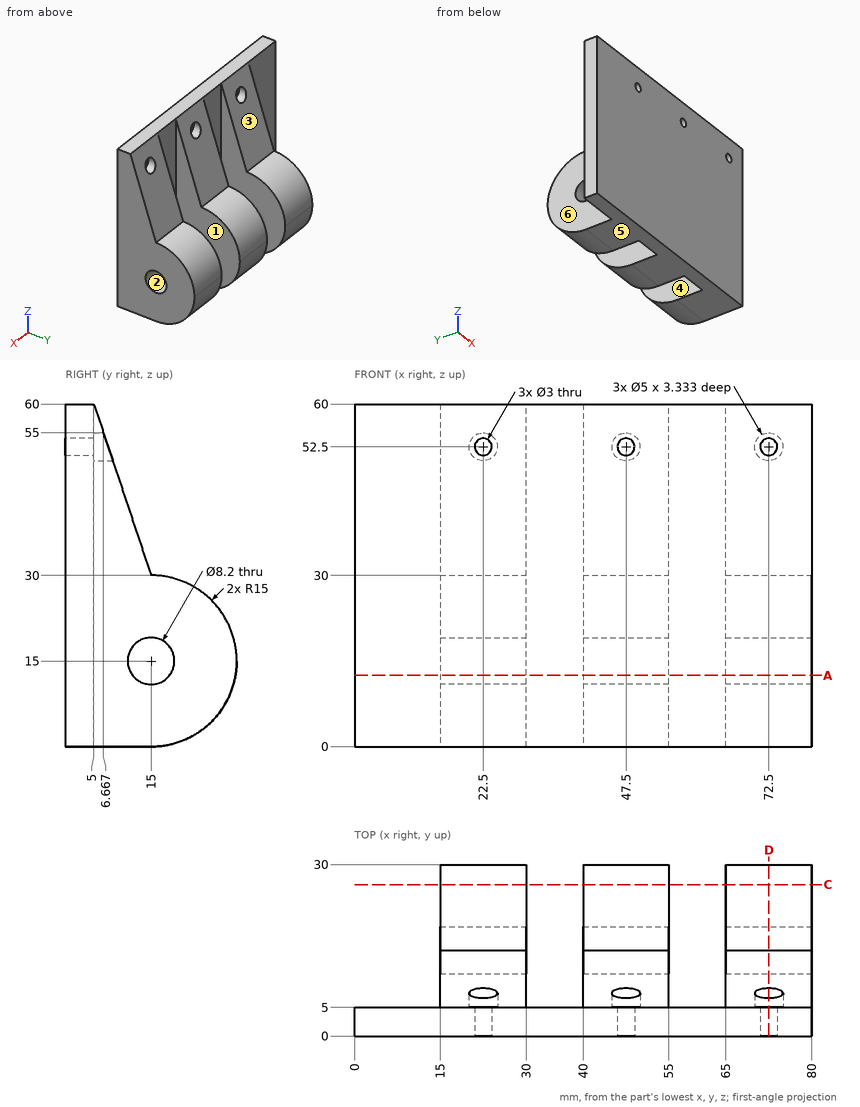
Study the drawing (mm; zero at the part's minimum x, y, z) and answer. A direction names the side the tool comes from. Give positions to 0.01 mm unless a question says otherwise; leave off trailing zeros. Write each loop counter-clockwise with the first axis right and the second up, starting at its lowest first coordinate (ties: lowest second). Pieces come first, ordered by that corner, then holes. Notation, with made-up numbers: M 88,12.25 L 117,12.25 A16 cw 117,35.25 Z; hole C 53.25,22.25 d8. An arc over 180 degrees is marked long. Put each result on its own line as item: value. Start each with the question number.
1. The part is cut by section D-D, the plane x = 72.5. Give the number of separate pieces and of enclosed holes in the cut face, and give its area (3 significant figures).
2. The part is cut by section C-C, the plane y = 26.5. Give the vertices of the cut face in (x, z).
3. Consider line 1 along X through (y, z) = (5.5, 48); line 2 along Y through (x, z) = (19.5, 15); line 3 along Z through (x, y) = (72.5, 2.65). Determine where each line is inside the solid, lowest interval first.
4. For a pull along Z with two mould halves and no side action, classify the marked faces 1, 2 and 3 as released by +Z, released by -Z, zero draft, split by the parting line, or undercut.
5. Which of the six approach directions +Z, -Z, +X, -X, +Y, -Y give full straight-line access (tool end or side, diameter ignored) to the marked faces 4, 5 and 6?
6. The part is cut by section A-A, the plane z = 12.5. Give the vertices of the cut face in (x, y).
7. Each of these flat-tipped pins is pushed along its axis until it touches: pin 1 Ø5 at (y, z) = (15, 15) entering from -X; pin 2 Ø1 at (x, y) = (22, 15.5) entering from -Z; pin 3 Ø4.5 at (x, z) = (47.5, 52.5) entering from +Y; pin 4 Ø4 at (x, z) = (16.5, 45.5) entering from +Y. Where does it stop, or does it pass through?
Final values:
1. separate pieces: 2
1. enclosed holes: 1
1. area: 1,020 mm²
2. outline: M 15,5.37 L 30,5.37 L 30,24.63 L 15,24.63 Z; M 40,5.37 L 55,5.37 L 55,24.63 L 40,24.63 Z; M 65,5.37 L 80,5.37 L 80,24.63 L 65,24.63 Z
3. line 1: x = 15 to 30, 40 to 55, 65 to 80
3. line 2: y = 0 to 10.9, 19.1 to 30
3. line 3: z = 0 to 51, 54 to 60
4. face 1: zero draft
4. face 2: undercut
4. face 3: released by +Z
5. face 4: +Z, -Z, +Y
5. face 5: -Z, +X, -X, +Y, -Y
5. face 6: +Z, -Z, -X, +Y
6. outline: M 0,0 L 80,0 L 80,11.75 L 65,11.75 L 65,5 L 55,5 L 55,11.75 L 40,11.75 L 40,5 L 30,5 L 30,11.75 L 15,11.75 L 15,5 L 0,5 Z; M 15,18.25 L 30,18.25 L 30,29.79 L 15,29.79 Z; M 40,18.25 L 55,18.25 L 55,29.79 L 40,29.79 Z; M 65,18.25 L 80,18.25 L 80,29.79 L 65,29.79 Z
7. pin 1: passes through
7. pin 2: stops at z = 0
7. pin 3: stops at y = 5
7. pin 4: stops at y = 10.5
